from build123d import *

# Parameters (mm, degrees)
SKETCH1_W           = 180
SKETCH1_H           = 104
BOSS_EXTRUDE1_DEPTH = 6.2
BOSS_EXTRUDE2_START = 5
SKETCH3_W           = 6.2
SKETCH3_H           = 15
BOSS_EXTRUDE2_DEPTH = 170


with BuildPart() as part:
    # Sketch1 → Boss-Extrude1 (new body)
    with BuildSketch(Plane(origin=(0, 0, 0), x_dir=(1, 0, 0), z_dir=(0, 1, 0))):
        Rectangle(SKETCH1_W, SKETCH1_H)
    extrude(amount=BOSS_EXTRUDE1_DEPTH)

    # Sketch3 → Boss-Extrude2 (add)
    with BuildSketch(Plane.ZY.offset(-90).offset(BOSS_EXTRUDE2_START)):
        with Locations((46.1, -7.5)):
            Rectangle(SKETCH3_W, SKETCH3_H)
        Polygon((36.3, -6.8), (27.5, -6.8), (27.5, 0), (21.3, 0), (21.3, -13), (36.3, -13), align=None)
        Polygon((-21.3, -13), (-21.3, 0), (-27.5, 0), (-27.5, -6.8), (-36.3, -6.8), (-36.3, -13), align=None)
        with Locations((-46.1, -7.5)):
            Rectangle(SKETCH3_W, SKETCH3_H)
    extrude(amount=BOSS_EXTRUDE2_DEPTH)


solid = part.part
Can you work these out from the model? Positions are in its coordinate system, mm. A direction names the side the tool comes from. Give positions to 0.01 mm unless a question says otherwise; leave off trailing zeros. Order: outer loops, then holes, each group sorted by start corner. A loop starts at its lowest first (then second) coordinate and runs counter-clockwise, first axis right, second up. Notation, with made-up numbers: M -3.75,60.25 L 54.25,60.25 A23 ccw 54.25,93.25 Z; hole C 84,0.5 d2. An arc over 180 degrees is marked long. Use a Markdown table: item, result. Add a question column.
Item 1: Will these pins go through, and if not, where does the flat tip stop? pin 1 (16.5 mm diameter, centred on x = -5, z = 25, fed in from -Y); pin 2 (2 mm diameter, centred on x = -35.5, y = -3, fed in from +Z); pin 3 (6 mm diameter, centred on y = -12.5, z = -24, fed in from -X).
Item 2: Suppose I cut it at C-C (x = 77.5). List the corners of the cut face in (y, z) for me.
Item 3: We'd pull the mould along Z, two halves only. Please class faces 5 (the flat face through (-90, 3, 1)), 6 (the flat face through (1, -8, -49.2)), 7 (the flat face through (1, -13, 29)), 8 (the flat face through (-1, 0, -1)): +Z half, -Z half, draft (parallel to the pull), parting line (faces both ways), or undercut.
Item 4: For faces 1 (the flat face through (85, -7, 46)), 2 (the flat face through (-85, -8, -27)), 3 (the flat face through (1, -3, -27.5)), 4 (the flat face through (1, -7, -21.3)), which set-ups out of +Z, -Z, +X, -X, +Y, -Y let a thin tool reach every point of the face, with its end or its side?
Item 5: Suppose I cut it at A-A (y = -2). List the corners of the cut face in (x, z) for me.
Item 6: If I drill on L1, parallel to Z at x = -61, y = -2.5; L2, parallel to Z at x = -74, y = -12; L3, parallel to Y at x = -38, z = 35, over which ranges is the centre line in solid material (lowest first)? Write a range as [from, to].
Item 7: Suppose I cut it at B-B (z = -34). List the corners of the cut face in (x, y) for me, then the cut area to 3 significant figures.
Item 8: Suppose I cut it at D-D (z = -45). List the corners of the cut face in (x, y) for me.
Answer sheet:
| question | item | result |
|---|---|---|
| 1 | pin 1 | stops at y = -13 |
| 1 | pin 2 | stops at z = 49.2 |
| 1 | pin 3 | stops at x = -85 |
| 2 | outline | M -15,-49.2 L 0,-49.2 L 0,-52 L 6.2,-52 L 6.2,52 L 0,52 L 0,49.2 L -15,49.2 L -15,43 L 0,43 L 0,27.5 L -6.8,27.5 L -6.8,36.3 L -13,36.3 L -13,21.3 L 0,21.3 L 0,-21.3 L -13,-21.3 L -13,-36.3 L -6.8,-36.3 L -6.8,-27.5 L 0,-27.5 L 0,-43 L -15,-43 Z |
| 3 | face 5 | draft |
| 3 | face 6 | -Z half |
| 3 | face 7 | undercut |
| 3 | face 8 | undercut |
| 4 | face 1 | +Z, -Z, +X, -Y |
| 4 | face 2 | +Z, -Z, -X, -Y |
| 4 | face 3 | +X, -X |
| 4 | face 4 | +X, -X, -Y |
| 5 | outline | M -85,-49.2 L 85,-49.2 L 85,-43 L -85,-43 Z; M -85,-27.5 L 85,-27.5 L 85,-21.3 L -85,-21.3 Z; M -85,21.3 L 85,21.3 L 85,27.5 L -85,27.5 Z; M -85,43 L 85,43 L 85,49.2 L -85,49.2 Z |
| 6 | L1 | z = [-49.2, -43], [-27.5, -21.3], [21.3, 27.5], [43, 49.2] |
| 6 | L2 | z = [-49.2, -43], [-36.3, -21.3], [21.3, 36.3], [43, 49.2] |
| 6 | L3 | y = [-13, -6.8], [0, 6.2] |
| 7 | outline | M -90,0 L 90,0 L 90,6.2 L -90,6.2 Z; M -85,-13 L 85,-13 L 85,-6.8 L -85,-6.8 Z |
| 7 | area | 2,170 mm² |
| 8 | outline | M -90,0 L -85,0 L -85,-15 L 85,-15 L 85,0 L 90,0 L 90,6.2 L -90,6.2 Z |
